Could you check a few things on this drawing? It's one solid part, dimensions in mm from its lowest x, y, z. Give positions to 0.01 mm unless a question says otherwise; leave off trailing zeros. Order: outer loops, then holes, each group sorted by start corner. A loop starts at its lowest first (then second) coordinate and runs counter-clockwise, first axis right, second up.
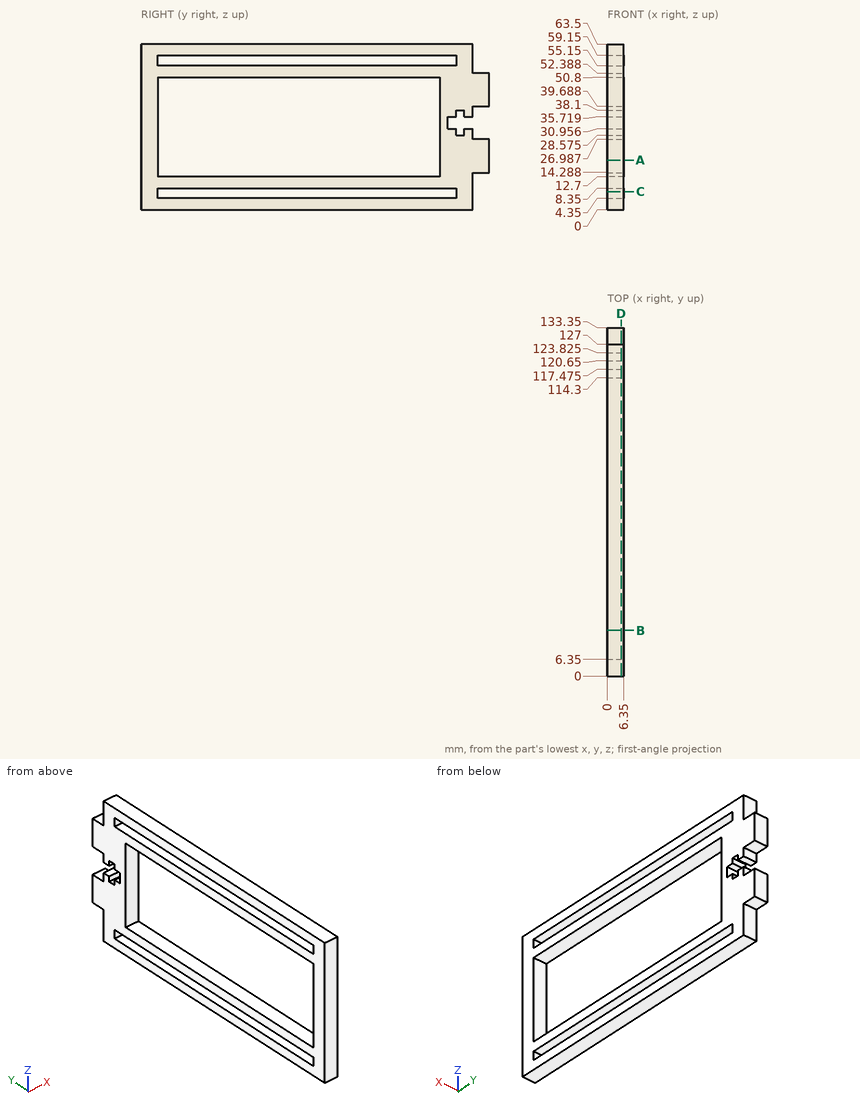
1) If I drill on line 1 (Z direction, x = 3.5, y = 9); line 2 (Y direction, x = 2.25, z = 25); line 3 (Y direction, x = 4.5, z = 5), over which ranges is the centre line in solid material (lowest first)?
2) I'm going to push flat-ended pins straight in: pin 1 Ø3 at (x, y) = (2.5, 130.5) entering from -Z; pin 2 Ø1.9 at (x, z) = (3.5, 60.5) entering from +Y. Where does each tip first touch, or does it pass through?
3) Suppose I cut it at D-D (x = 5.25). Give the number of separate pieces and of enclosed holes in the cut face, and give its area (3 significant figures).
4) Suppose I cut it at B-B (y = 17.5). Please give me the cut outline in (x, z).
5) Suppose I cut it at C-C (z = 7). Please give me the cut outline in (x, y).
6) Suppose I cut it at A-A (z = 19). Please give me the cut outline in (x, y).
Results:
1. line 1: z = 0 to 4.35, 8.35 to 12.7, 50.8 to 55.15, 59.15 to 63.5
1. line 2: y = 0 to 6.35, 114.3 to 133.35
1. line 3: y = 0 to 6.35, 120.65 to 127
2. pin 1: stops at z = 14.29
2. pin 2: stops at y = 127
3. separate pieces: 1
3. enclosed holes: 3
3. area: 3,140 mm2
4. outline: (0, 0) - (6.35, 0) - (6.35, 4.35) - (0, 4.35) - close; (0, 8.35) - (6.35, 8.35) - (6.35, 12.7) - (0, 12.7) - close; (0, 50.8) - (6.35, 50.8) - (6.35, 55.15) - (0, 55.15) - close; (0, 59.15) - (6.35, 59.15) - (6.35, 63.5) - (0, 63.5) - close
5. outline: (0, 0) - (6.35, 0) - (6.35, 6.35) - (0, 6.35) - close; (0, 120.65) - (6.35, 120.65) - (6.35, 127) - (0, 127) - close
6. outline: (0, 0) - (6.35, 0) - (6.35, 6.35) - (0, 6.35) - close; (0, 114.3) - (6.35, 114.3) - (6.35, 133.35) - (0, 133.35) - close
